Source: CAD feature listing. Evaluate the final solid. Frame: model axes, mm. A direction names the side the tool comes from. Give positions to 0.01 mm unless a question says otherwise; leave off trailing zeros. Loops run counter-clockwise (first coordinate to the right, second up) from the corner with the lowest first, then second, coordinate; pieces in that order, holes last.
```python
from build123d import *

# Parameters (mm, degrees)
EXTRUDE_1_DEPTH          = 30
SKETCH_3_R               = 2.65
EXTRUDE_2_DEPTH          = 15
SKETCH_4_R               = 5
CUT_EXTRUDE_1_DEPTH      = 5
CUT_EXTRUDE_2_DEPTH      = 3
CUT_EXTRUDE_3_DEPTH      = 47.097722286
CUT_EXTRUDE_3_DEPTH_BACK = 47.097722286
SKETCH_6_R               = 1.7
FILLET_1_R               = 2
FILLET_2_R               = 1
FILLET_3_R               = 1
FILLET_5_R               = 2


with BuildPart() as part:
    # 草图2 → 凸台-拉伸1 (new body)
    with BuildSketch(Plane.XY):
        Polygon((0, 0), (0, 2.8), (11, 2.8), (11, 8.2), (0, 8.2), (0, 11), (16, 11), (16, 0), align=None)
    extrude(amount=-EXTRUDE_1_DEPTH)

    # 草图3 → 凸台-拉伸2 (add)
    with BuildSketch(Plane.XY):
        with BuildLine():
            Line((9.5, 11), (9.5, 16.732173124))
            ThreePointArc((9.5, 16.732173124), (20.711715487, 31.625310339), (22.5, 13.06971445))
            Line((22.5, 13.06971445), (22.5, 11.258330249))
            Line((22.5, 11.258330249), (16, 0))
            Line((16, 0), (16, 11))
            Line((16, 11), (9.5, 11))
        make_face()
        with Locations((18, 22)):
            Circle(SKETCH_3_R, mode=Mode.SUBTRACT)
    extrude(amount=-EXTRUDE_2_DEPTH)

    # 草图4 → 切除-拉伸1 (cut)
    with BuildSketch(Plane(origin=(0, 0, -15), x_dir=(-1, 0, 0), z_dir=(0, 0, -1))):
        with Locations((-18, 22)):
            Circle(SKETCH_4_R)
    extrude(amount=-CUT_EXTRUDE_1_DEPTH, mode=Mode.SUBTRACT)

    # 草图5 → 切除-拉伸2 (cut)
    with BuildSketch(Plane.XY):
        Polygon((18, 26.792007234), (13.85, 24.396003617), (13.85, 19.603996383), (18, 17.207992766), (22.15, 19.603996383), (22.15, 24.396003617), align=None)
    extrude(amount=-CUT_EXTRUDE_2_DEPTH, mode=Mode.SUBTRACT)

    # 草图6 → 切除-拉伸3 (cut, two sides: drawn at the far end of the back side and taken through both)
    with BuildSketch(Plane(origin=(0, 11, 0), x_dir=(1, 0, 0), z_dir=(0, 1, 0)).offset(-CUT_EXTRUDE_3_DEPTH_BACK)):
        with Locations(Location((5, 6, 0), (0, 0, 180))):
            Circle(SKETCH_6_R)
        with Locations(Location((5, 24, 0), (0, 0, 180))):
            Circle(SKETCH_6_R)
    extrude(amount=CUT_EXTRUDE_3_DEPTH + CUT_EXTRUDE_3_DEPTH_BACK, mode=Mode.SUBTRACT)

    # 圆角1
    fillet_1_edges = [part.edges().sort_by_distance(p)[0] for p in [
        (9.5, 11, -7.5),
    ]]
    fillet(fillet_1_edges, radius=FILLET_1_R)

    # 圆角2
    fillet_2_edges = [part.edges().sort_by_distance(p)[0] for p in [
        (9.5, 16.732173124, -7.5),
    ]]
    fillet(fillet_2_edges, radius=FILLET_2_R)

    # 圆角3
    fillet_3_edges = [part.edges().sort_by_distance(p)[0] for p in [
        (22.5, 13.06971445, -7.5),
        (22.5, 11.258330249, -7.5),
    ]]
    fillet(fillet_3_edges, radius=FILLET_3_R)

    # 圆角5
    fillet_5_edges = [part.edges().sort_by_distance(p)[0] for p in [
        (8, 0, 0),
        (8, 0, -30),
    ]]
    fillet(fillet_5_edges, radius=FILLET_5_R)


solid = part.part
```
(1) Mould query, pull axis X, two halves, no side actions, for faces 1 (the flat face through (16, 6, -22)), 2 (the cylindrical face through (8.46, 0.6, -0.57)), 3 (the cylindrical face through (5.221, 9.58, -22.314)), 4 (the cylindrical face through (5.221, 1.38, -22.314)). Classes: pulls with the +X half, pulls with the -X half, needs draft (parallel to the pull), parting line crosses it, or undercut.
A:
face 1: pulls with the +X half
face 2: needs draft
face 3: undercut
face 4: undercut
(2) Reachability of faces 5 (the flat face through (15.95, 25.61, -1.48)), 6 (the flat face through (6, 11, -18)), 7 (the flat face through (0, 1, -15)), 8 (the flat face through (11, 5, -15)), 9 (the flat face through (22.5, 12, -7)) from +Z, -Z, +X, -X, +Y, -Y: full face, straight path, thin tool, end or side. Return the list, or none.
A:
face 5: +Z
face 6: -Z, -X, +Y
face 7: +Z, -Z, -X, +Y, -Y
face 8: +Z, -Z, -X
face 9: +Z, -Z, +X, -Y
(3) Section A-A, the plane z = -6. Return the cut outline in (x, y).
A:
outline: (0, 0) - (3.3, 0) - (3.3, 2.8) - (0, 2.8) - close; (0, 8.2) - (3.3, 8.2) - (3.3, 11) - (0, 11) - close; (6.7, 0) - (16, 0) - (22.37, 11.03) arc R1 ccw to (22.5, 11.53) - (22.5, 12.47) arc R1 cw to (23, 13.34) arc R10 ccw (long way) to (9.36, 16.96) arc R1 cw to (9.5, 16.45) - (9.5, 13) arc R2 cw to (7.5, 11) - (6.7, 11) - (6.7, 8.2) - (11, 8.2) - (11, 2.8) - (6.7, 2.8) - close; hole circle Ø5.3 at (18, 22)
(4) Section B-B, the plane y = 22. Return the cut outline in (x, z).
A:
outline: (8, -15) - (13, -15) - (13, -10) - (15.35, -10) - (15.35, -3) - (13.85, -3) - (13.85, 0) - (8, 0) - close; (20.65, -10) - (23, -10) - (23, -15) - (28, -15) - (28, 0) - (22.15, 0) - (22.15, -3) - (20.65, -3) - close
(5) Section C-C, the plane x = 5. Return the cut outline in (y, z), then the cut area to 3 significant figures.
A:
outline: (0, -28) arc R2 ccw to (2, -30) - (2.8, -30) - (2.8, -25.7) - (0, -25.7) - close; (0, -22.3) - (2.8, -22.3) - (2.8, -7.7) - (0, -7.7) - close; (0, -4.3) - (2.8, -4.3) - (2.8, 0) - (2, 0) arc R2 ccw to (0, -2) - close; (8.2, -30) - (11, -30) - (11, -25.7) - (8.2, -25.7) - close; (8.2, -22.3) - (11, -22.3) - (11, -7.7) - (8.2, -7.7) - close; (8.2, -4.3) - (11, -4.3) - (11, 0) - (8.2, 0) - close
area: 128 mm2
(6) First-contact query: pin 1 (5.5 mm diameter, centred on x = 5, z = -24, fed in from +Y); pin 2 (5 mm diameter, centred on x = 15.5, y = 21.5, fed in from -Z); pin 3 (8 mm diameter, centred on y = 27.5, z = -5, fed in from -X). Flat tips, straight axial feed; report the tip coordinate or a pass-through.
A:
pin 1: stops at y = 11
pin 2: stops at z = -15
pin 3: stops at x = 8.11
(7) Ray query, line 1 along Z through (x, y) = (5, 1.4); line 2 along X through (y, z) = (9.5, -24); line 3 along Y through (x, z) = (7, -16.5). Return the intervals inside material, ascending.
A:
line 1: z = -29.91 to -25.7, -22.3 to -7.7, -4.3 to -0.09
line 2: x = 0 to 3.3, 6.7 to 16
line 3: y = 0 to 2.8, 8.2 to 11
(8) Section D-D, the plane z = -24. Return the cut outline in (x, y), then the cut area to 3 significant figures.
A:
outline: (0, 0) - (3.3, 0) - (3.3, 2.8) - (0, 2.8) - close; (0, 8.2) - (3.3, 8.2) - (3.3, 11) - (0, 11) - close; (6.7, 0) - (16, 0) - (16, 11) - (6.7, 11) - (6.7, 8.2) - (11, 8.2) - (11, 2.8) - (6.7, 2.8) - close
area: 97.6 mm2
